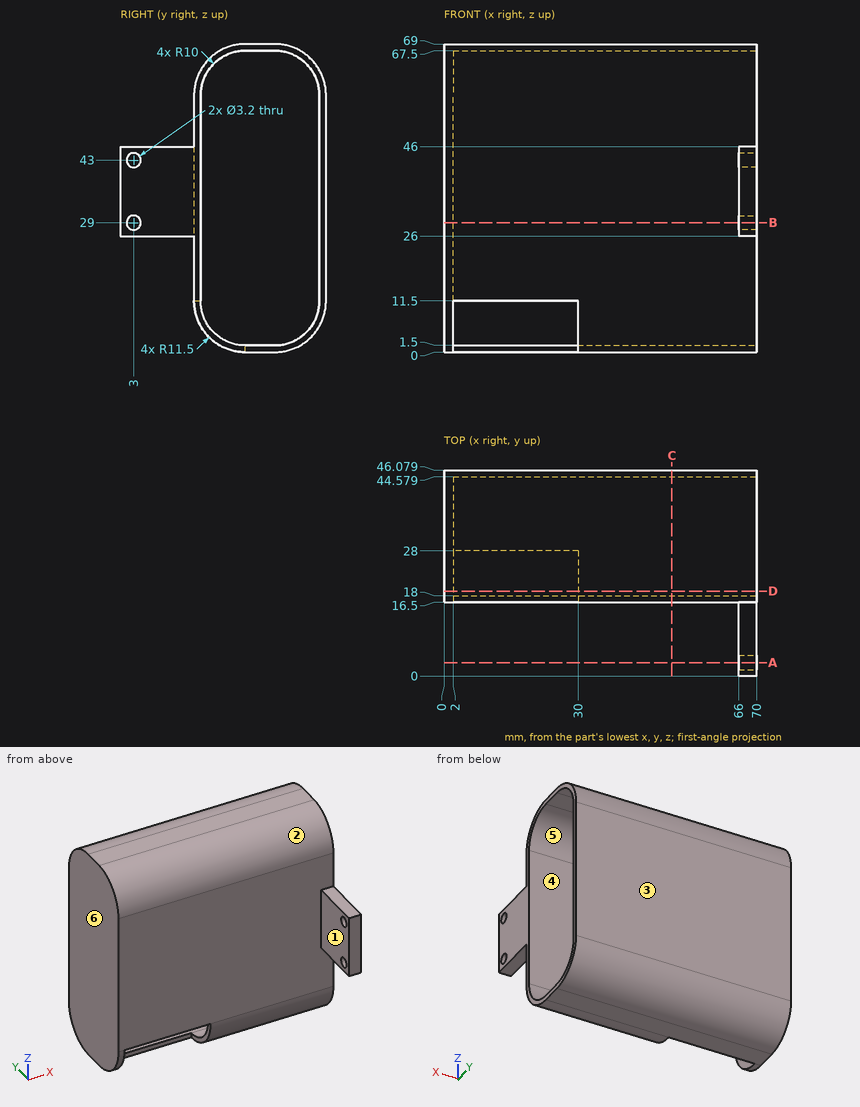
For this review, use the dimensioned drawing (mm, ordinates from the lowest corner) and the shaded views. A direction names the side the tool comes from. Coordinates: 2 decimals unless noted, no trailing zeros. Loops run counter-clockwise (first coordinate to the right, second up) from the corner with the lowest first, then second, coordinate; pieces in that order, holes last. Notation, with made-up numbers: (19, 82.25) -> (32, 82.25) arc R37 cw to (32, 120.25) -> close; hole circle Ø4 at (-29.5, -12.5). An arc over 180 degrees is marked (long way). Use a Markdown table: item, result. Add a question column.
Item 1: We need section C-C, the plane x = 51. Write out the cut boundary in (y, z).
Item 2: We need section D-D, the plane y = 19. Write out the cut boundary in (x, z), and give its area (3 significant figures).
Item 3: Clearance check with flat-ended pins moving along their axes: P1, Ø14, axis at y = 30, z = 21.5, coming from the +X side; P2, Ø4, axis at x = 56.5, z = 27, coming from the -Y side; P3, Ø8, axis at x = 52, y = 18.5, coming from the +Z side. State where each tip first meets the part, or that it passes through.
Item 4: The part is to be moulded in two halves that separate along Y. For the marked faces 3, 4, 5 and 6, say which applies: +Y half, -Y half, draft (parallel to the pull), parting line (faces both ways), or undercut.
Item 5: Machinability: for the marked faces 1 and 2, which of the approach directions +Z, -Z, +X, -X, +Y, -Y give a long, thin tool a straight path to every point of the face, cutting with its end or side? Answer none if there is none.
Item 6: We need section B-B, the plane z = 29. Write out the cut boundary in (x, y).
Item 7: Wall thickness on L1, parallel to Y at x = 68.95, z = 43; L2, parallel to Y at x = 11.5, z = 28.5; L3, parallel to Z at x = 61.5, y = 31: over which ranges is each line inside the solid? List them lowest first. Write a range as from..to.
Item 8: We need section A-A, the plane y = 3. Write out the cut boundary in (x, z), and give its area (3 significant figures).
Numbers:
| question | item | result |
|---|---|---|
| 1 | outline | (16.5, 11.5) arc R11.5 ccw to (28, 0) -> (34.58, 0) arc R11.5 ccw to (46.08, 11.5) -> (46.08, 57.5) arc R11.5 ccw to (34.58, 69) -> (28, 69) arc R11.5 ccw to (16.5, 57.5) -> close; hole (18, 11.5) arc R10 ccw to (28, 1.5) -> (34.58, 1.5) arc R10 ccw to (44.58, 11.5) -> (44.58, 57.5) arc R10 ccw to (34.58, 67.5) -> (28, 67.5) arc R10 ccw to (18, 57.5) -> close |
| 2 | outline | (0, 4.34) -> (2, 4.34) -> (2, 61.86) -> (70, 61.86) -> (70, 64.66) -> (0, 64.66) -> close; (30, 4.34) -> (70, 4.34) -> (70, 7.14) -> (30, 7.14) -> close |
| 2 | area | 423 mm^2 |
| 3 | P1 | stops at x = 2 |
| 3 | P2 | stops at y = 16.5 |
| 3 | P3 | stops at z = 67.6 |
| 4 | face 3 | +Y half |
| 4 | face 4 | undercut |
| 4 | face 5 | undercut |
| 4 | face 6 | draft |
| 5 | face 1 | +Z, -Z, -X, -Y |
| 5 | face 2 | +Z, +X, -X, -Y |
| 6 | outline | (0, 16.5) -> (66, 16.5) -> (66, 4.6) -> (70, 4.6) -> (70, 18) -> (2, 18) -> (2, 44.58) -> (70, 44.58) -> (70, 46.08) -> (0, 46.08) -> close; (66, 0) -> (70, 0) -> (70, 1.4) -> (66, 1.4) -> close |
| 7 | L1 | y = 0..1.4, 4.6..18, 44.58..46.08 |
| 7 | L2 | y = 16.5..18, 44.58..46.08 |
| 7 | L3 | z = 0..1.5, 67.5..69 |
| 8 | outline | (66, 26) -> (70, 26) -> (70, 27.4) -> (66, 27.4) -> close; (66, 30.6) -> (70, 30.6) -> (70, 41.4) -> (66, 41.4) -> close; (66, 44.6) -> (70, 44.6) -> (70, 46) -> (66, 46) -> close |
| 8 | area | 54.4 mm^2 |
